The listing builds one solid part. Answer for the finished solid, in the listing's coordinates (mm). A direction names the side the tool comes from. Round coordinates to 2 decimals unless told otherwise and drop trailing zeros. Write each loop counter-clockwise with the first axis right and the second up, starting at its lowest first coordinate (ties: lowest second). Pieces come first, ordered by that corner, then holes. Notation, with made-up numbers: (76.5, 17) - (114.5, 17) arc R21 cw to (114.5, 21) - close; hole circle Ø5 at (14.25, 66.25). An arc over 180 degrees is marked (long way). Return JSON: item names as keys, results as strings. Group by question number.
(1) Section C-C, the plane y = 15.75 is taken. Write down the section's boundary in (x, z).
(2) Each of these flat-tipped pins is pushed along its axis until it touches: pin 1 (10 mm diameter, centred on y = 18, z = -23.5, fed in from +X); pin 2 (8 mm diameter, centred on y = 23, z = -1, fed in from +X); pin 3 (10 mm diameter, centred on x = -3.5, z = 24, fed in from -Y); pin 4 (0.7 mm diameter, centred on x = 0.5, z = 23.5, fed in from +Y). Where does it stop, or does it pass through?
(3) Section D-D, the plane z = -8 is taken. Write down the section's boundary in (x, y), then the cut area to 3 significant figures.
(4) Find the intervals of material crossed by line 1 along Y through (x, z) = (4, -15); line 2 along X through (y, z) = (13.25, -17); line 3 along X through (y, z) = (3.25, -19.5), in increasing order. Write a range as [from, to].
(5) Which of the six approach directions +Z, -Z, +X, -X, +Y, -Y give full straight-line access (tool end or side, diameter ignored) to faces 1 (the cylindrical face through (9.15, 16.7, -21.4)), 2 (the cylindrical face through (-9.15, 2.1, -21.4)), 3 (the flat face through (10, 2, -10.25))?
(6) Section B-B, the plane x = 0 is taken. Write down the section's boundary in (y, z).
(7) Section A-A, the plane z = -23 is taken. Write down the section's boundary in (x, y).
```python
from build123d import *

# Parameters (mm, degrees)
SKETCH_1_W          = 22.3
SKETCH_1_H          = 64.5
EXTRUDE_1_DEPTH     = 18.8
SKETCH_2_R          = 2.7
EXTRUDE_2_DEPTH     = 9.1
SKETCH_3_W          = 7.709030296
SKETCH_3_H          = 1.42648476
SKETCH_3_H_2        = 1.599270141
CUT_EXTRUDE_1_DEPTH = 8
CUT_EXTRUDE_2_DEPTH = 22


with BuildPart() as part:
    # 草图1 → 凸台-拉伸1 (new body)
    with BuildSketch(Plane(origin=(0, 0, 0), x_dir=(1, 0, 0), z_dir=(0, 1, 0))):
        Rectangle(SKETCH_1_W, SKETCH_1_H)
    extrude(amount=EXTRUDE_1_DEPTH)

    # 草图2 → 凸台-拉伸2 (add)
    with BuildSketch(Plane(origin=(0, 18.8, 0), x_dir=(1, 0, 0), z_dir=(0, 1, 0))):
        with Locations(Location((0, -20.97, 0), (0, 0, 270))):
            Circle(SKETCH_2_R)
    extrude(amount=EXTRUDE_2_DEPTH)

    # 草图3 → 切除-拉伸1 (cut)
    with BuildSketch(Plane(origin=(0, 27.9, 0), x_dir=(1, 0, 0), z_dir=(0, 1, 0))):
        with Locations((0, -18.40675762)):
            Rectangle(SKETCH_3_W, SKETCH_3_H)
        with Locations((0, -23.619635071)):
            Rectangle(SKETCH_3_W, SKETCH_3_H_2)
    extrude(amount=-CUT_EXTRUDE_1_DEPTH, mode=Mode.SUBTRACT)

    # 草图4 → 切除-拉伸2 (cut)
    with BuildSketch(Plane(origin=(0, 0, -32.25), x_dir=(-1, 0, 0), z_dir=(0, 0, -1))):
        with BuildLine():
            ThreePointArc((11.15, 7), (9.099747468, 2.050252532), (4.15, 0))
            Line((4.15, 0), (11.15, 0))
            Line((11.15, 0), (11.15, 7))
        make_face()
        with BuildLine():
            ThreePointArc((4.15, 18.8), (9.099747468, 16.749747468), (11.15, 11.8))
            Line((11.15, 11.8), (11.15, 18.8))
            Line((11.15, 18.8), (4.15, 18.8))
        make_face()
        with BuildLine():
            Line((-11.15, 0), (-4.15, 0))
            ThreePointArc((-4.15, 0), (-9.099747468, 2.050252532), (-11.15, 7))
            Line((-11.15, 7), (-11.15, 0))
        make_face()
        with BuildLine():
            Line((-11.15, 18.8), (-11.15, 11.8))
            ThreePointArc((-11.15, 11.8), (-9.099747468, 16.749747468), (-4.15, 18.8))
            Line((-4.15, 18.8), (-11.15, 18.8))
        make_face()
    extrude(amount=-CUT_EXTRUDE_2_DEPTH, mode=Mode.SUBTRACT)


solid = part.part
```
Working result:
{
 "1": {"outline": "(-11.15, -10.25) - (-9.93, -10.25) - (-9.93, -32.25) - (9.93, -32.25) - (9.93, -10.25) - (11.15, -10.25) - (11.15, 32.25) - (-11.15, 32.25) - close"},
 "2": {"pin 1": "stops at x = 11.05", "pin 2": "passes through", "pin 3": "stops at y = 0", "pin 4": "stops at y = 19.9"},
 "3": {"outline": "(-11.15, 0) - (11.15, 0) - (11.15, 18.8) - (-11.15, 18.8) - close", "area": "419 mm^2"},
 "4": {"line 1": "y = [0, 18.8]", "line 2": "x = [-11, 11]", "line 3": "x = [-10.06, 10.06]"},
 "5": {"face 1": "-Z, +X, +Y", "face 2": "-Z, -X, -Y", "face 3": "-Z, +X, -Y"},
 "6": {"outline": "(0, -32.25) - (18.8, -32.25) - (18.8, 18.27) - (19.9, 18.27) - (19.9, 19.12) - (27.9, 19.12) - (27.9, 22.82) - (19.9, 22.82) - (19.9, 23.67) - (18.8, 23.67) - (18.8, 32.25) - (0, 32.25) - close"},
 "7": {"outline": "(-11.15, 7) arc R7 ccw to (-4.15, 0) - (4.15, 0) arc R7 ccw to (11.15, 7) - (11.15, 11.8) arc R7 ccw to (4.15, 18.8) - (-4.15, 18.8) arc R7 ccw to (-11.15, 11.8) - close"}
}
